```python
from build123d import *

# Parameters (mm, degrees)
F1_DEPTH = 76.2
F2_DEPTH = 25.4
F3_R     = 11.245644
F4_DEPTH = 152.4


with BuildPart() as f1:
    # F0 (on Front) → F1 (new body)
    with BuildSketch(Plane.XZ):
        Polygon((0, 41.862), (0, 0), (90.346729, 0), (38.561046, 41.862), align=None)
    extrude(amount=F1_DEPTH)

    # F0 (on Front) → F2 (join)
    with BuildSketch(Plane.XZ):
        Polygon((0, 41.862), (0, 0), (90.346729, 0), (38.561046, 41.862), align=None)
        Polygon((0, 55.065785), (0, 41.862), (38.561046, 41.862), (90.346729, 0), (106.680565, 0), (38.561046, 55.065785), align=None)
    extrude(amount=F2_DEPTH)

    # F3 (on Right) → F4 (cut)
    with BuildSketch(Plane.YZ):
        with Locations((-50.974112, 21.47734)):
            Circle(F3_R)
    extrude(amount=F4_DEPTH, mode=Mode.SUBTRACT)


solid = f1.part
```
For this review, take the finished solid that the model builds, in its own axes (mm). A direction names the side the tool comes from. Coordinates: 2 decimals unless noted, no trailing zeros. Loops run counter-clockwise (first coordinate to the right, second up) from the corner with the lowest first, then second, coordinate; pieces in that order, holes last.
1. Add section A-A, the plane z = 27. Give the boundary of the cut face in (x, y).
2. For line 1 (Y direction, x = 14.5, z = 44.5); line 2 (Y direction, x = 53, z = 28); line 3 (Y direction, x = 39, z = 20), list the stretches that pass through material, from the lowest coordinate up.
3. Add section C-C, the plane x = 7. Give the boundary of the cut face in (y, z), then the cut area to 3 significant figures.
4. Add section B-B, the plane y = -57. Give the boundary of the cut face in (x, z), then the cut area to 3 significant figures.
5. Add section D-D, the plane x = 73. Give the boundary of the cut face in (y, z).
6. For faces 5 (the flat face through (73.098, -12.522, 27.147)), 6 (the flat face through (20, -50, 41.862)), list the 3-axis set-ups (+Z, -Z, +X, -X, +Y, -Y) from which the entire face can be reached by the end or side of a thin tool; tool diameter is ignored.
7. Insertion check: P1, Ø2, axis at y = -30, z = 24.5, coming from the +X side; P2, Ø3, axis at x = 38, y = -39.5, coming from the +Z side; P3, Ø6, axis at x = 80.5, y = -27.5, coming from the +Z side. Each pin has a flat end and moves straight along its axis. Give the tip position at first contact, or say it passes through.
8. Mouldability with a two-part tool opening along Z and no side actions: class faces 1 (the cylindrical face through (29.67, -53.41, 10.5)), 2 (the flat face through (64.816, -39.156, 20.638)), 3 (the flat face through (53, -38, 0)), 4 (the flat face through (49, -25.4, 34)) as +Z half, -Z half, draft (parallel to the pull), parting line (faces both ways), or undercut.
Result:
1. outline: (0, -76.2) - (56.95, -76.2) - (56.95, -60.77) - (0, -60.77) - close; (0, -41.18) - (56.95, -41.18) - (56.95, -25.4) - (73.28, -25.4) - (73.28, 0) - (0, 0) - close
2. line 1: y = -25.4 to 0
2. line 2: y = -76.2 to -60.13, -41.81 to 0
2. line 3: y = -76.2 to -62.12, -39.83 to 0
3. outline: (-76.2, 0) - (0, 0) - (0, 55.07) - (-25.4, 55.07) - (-25.4, 41.86) - (-76.2, 41.86) - close; hole circle Ø22.49 at (-50.97, 21.48)
3. area: 3,130 mm2
4. outline: (0, 0) - (90.35, 0) - (75.52, 11.98) - (0, 11.98) - close; (0, 30.97) - (52.03, 30.97) - (38.56, 41.86) - (0, 41.86) - close
4. area: 1,490 mm2
5. outline: (-76.2, 0) - (0, 0) - (0, 27.23) - (-25.4, 27.23) - (-25.4, 14.02) - (-42.55, 14.02) arc R11.25 cw to (-59.39, 14.02) - (-76.2, 14.02) - close
6. face 5: +Z, +X, +Y, -Y
6. face 6: +Z, +X, -X, -Y
7. P1: stops at x = 61.28
7. P2: stops at z = 41.86
7. P3: stops at z = 22.9
8. face 1: undercut
8. face 2: +Z half
8. face 3: -Z half
8. face 4: draft
